Autodesk Inventor part; units mm, degrees
ref_plane "YZ Plane" through (0, 0, 0) normal (1, 0, 0) x (0, 1, 0)
ref_plane "XZ Plane" through (0, 0, 0) normal (0, 1, 0) x (-1, 0, 0)
ref_plane "XY Plane" through (0, 0, 0) normal (0, 0, 1) x (1, 0, 0)
sketch "Sketch1" plane through (0, 0, 0) normal (0, 0, 1) x (1, 0, 0)
  line L0 (0, -3.175) -> (31.75, -3.175)
  line L1 (31.75, -3.175) -> (31.75, -28.575)
  line L2 (31.75, -28.575) -> (0, -28.575)
  line L3 (0, -28.575) -> (0, -3.175)
  line L4 (0, -3.175) -> (5.715, -3.175)
  line L5 (5.715, -3.175) -> (5.715, 15.875)
  line L6 (5.715, 15.875) -> (0, 15.875)
  line L7 (0, 15.875) -> (0, -3.175)
  line L8 (26.035, -3.175) -> (31.75, -3.175)
  line L9 (31.75, -3.175) -> (31.75, 15.875)
  line L10 (31.75, 15.875) -> (26.035, 15.875)
  line L11 (26.035, 15.875) -> (26.035, -3.175)
  point P0 (0, 0)
  dimension "d0" = 25.4
  dimension "d1" = 5.715
  dimension "d2" = 5.715
  dimension "d3" = 19.05
  dimension "d4" = 31.75
  dimension "d24" = 20.32
extrude "Extrusion1" add sketch "Sketch1" against normal blind 15.875
sketch "Sketch2" plane through (0, 0, 0) normal (0, 0, 1) x (1, 0, 0)
  line L0 (31.75, -28.575) -> (0, -28.575)
  circle A0 centre (15.875, -15.875) radius 8.7439
  dimension "d10" = 17.4879
  dimension "d13" = 12.7
extrude "Extrusion2" cut sketch "Sketch2" against normal blind 15.875
sketch "Sketch3" plane through (31.75, -3.175, 0) normal (1, 0, 0) x (0, 0, -1)
  line L0 (0, 19.05) -> (15.875, 19.05)
  line L1 (-0.1272, 19.05) -> (15.7478, 19.05)
  circle A0 centre (7.9375, 12.7) radius 2.4447
  dimension "d16" = 4.8895
  dimension "d17" = 6.35
  dimension "d18" = 0
extrude "Extrusion3" cut sketch "Sketch3" against normal through all
fillet "Fillet1" radius 1.5875 2 edges at (5.715, -3.175, -7.9375) (26.035, -3.175, -7.9375)
fillet "Fillet3" radius 6.35 2 edges at (0, -28.575, -7.9375) (31.75, -28.575, -7.9375)
sketch "Sketch5" plane through (0, 0, 0) normal (0, 0, 1) x (1, 0, 0)
  line L0 (31.75, 15.875) -> (31.75, -22.225)
  line L1 (0, -22.225) -> (0, 15.875)
  line L2 (0, -22.2885) -> (3.175, -22.2885)
  line L3 (3.175, -22.2885) -> (3.175, -9.4615)
  line L4 (3.175, -9.4615) -> (0, -9.4615)
  line L5 (0, -9.4615) -> (0, -22.2885)
  line L6 (31.75, -9.4615) -> (28.575, -9.4615)
  line L7 (28.575, -9.4615) -> (28.575, -22.2885)
  line L8 (28.575, -22.2885) -> (31.75, -22.2885)
  line L9 (31.75, -22.2885) -> (31.75, -9.4615)
  circle A0 centre (15.875, -15.875) radius 8.7439
  point P0 (0, 0)
  point P1 (3.175, -15.875)
  dimension "d33" = 12.827
  dimension "d34" = 3.175
  dimension "d35" = 3.175
  dimension "d41" = 0
extrude "Extrusion5" cut sketch "Sketch5" against normal blind 25.4 contours L0 L9 L8 L7 L6 | L1 L4 L3 L2 L5
sketch "Sketch6" plane through (0, 0, 0) normal (0, 0, 1) x (1, 0, 0)
  line L0 (0, -9.4615) -> (0, 15.875)
  line L1 (0, -9.4615) -> (3.175, -9.4615)
  circle A0 centre (2.8575, 3.2385) radius 1.5875
  circle A1 centre (28.8925, 3.2385) radius 1.5875
  line L2 (28.575, -9.4615) -> (31.75, -9.4615)
  line L3 (26.035, -1.5875) -> (26.035, 15.875)
  point P0 (0, 0)
  dimension "d42" = 3.175
  dimension "d43" = 2.8575
  dimension "d44" = 12.7
  dimension "d45" = 3.175
  dimension "d50" = 12.7
  dimension "d51" = 2.8575
extrude "Extrusion6" cut sketch "Sketch6" against normal blind 25.4
properties part number "Smaller Needle Bearing Mount" material "Polyethylene, High Density"
Here's how the part is built. I have some questions about the finished solid (model axes, mm). A direction names the side the tool comes from. Give positions to 0.01 mm unless a question says otherwise; leave off trailing zeros. Write each loop counter-clockwise with the first axis right and the second up, starting at its lowest first coordinate (ties: lowest second). Pieces come first, ordered by that corner, then holes.
(1) If I drill on L1, parallel to X at y = 9, z = -11 (3 decimals); L2, parallel to Y at x = 29, z = -9.25 (1 decimal); L3, parallel to X at y = -13, z = -12 (3 decimals), over which ranges is the centre line in solid material (lowest first)?
Output values:
L1: x = 0 to 5.715, 26.035 to 31.75
L2: y = -27.5 to -22.3, -9.5 to 1.7, 4.8 to 7.5, 11.6 to 15.9
L3: x = 3.175 to 7.617, 24.133 to 28.575
(2) Imagine slicing it at D-D, the plane y = 4. Write out the boundary of the cut face in (x, z) (3 decimals), and give its area (3 significant figures).
Output values:
outline: (0, -15.875) - (1.465, -15.875) - (1.465, 0) - (0, 0) - close; (4.25, -15.875) - (5.715, -15.875) - (5.715, 0) - (4.25, 0) - close; (26.035, -15.875) - (27.5, -15.875) - (27.5, 0) - (26.035, 0) - close; (30.285, -15.875) - (31.75, -15.875) - (31.75, 0) - (30.285, 0) - close
area: 93.0 mm2
(3) Imagine slicing it at A-A, the plane y = -1. Write out the boundary of the cut face in (x, z) (3 decimals), and give its area (3 significant figures).
Output values:
outline: (0, -15.875) - (5.715, -15.875) - (5.715, 0) - (0, 0) - close; (26.035, -15.875) - (31.75, -15.875) - (31.75, 0) - (26.035, 0) - close
area: 181 mm2
(4) On a 3-axis mill with a long thin cutter (end or side, diameter ignored), from which of +Z, -Z, +X, -X, +Y, -Y can I reach the whole of each face in a straight line? I mean faces 4 (the face through (6.19, -2.72, -8.05)), 5 (the face through (3.175, -16, -8)), 6 (the face through (28.575, -16, -8)). Say none if no direction works.
Output values:
face 4: +Z, -Z, +Y
face 5: +Z, -Z, -X
face 6: +Z, -Z, +X
(5) Will these pins go through, and if not, where does the flat tip stop? pin 1 (4 mm diameter, centred on y = -12.5, z = -4.5, fed in from -X) (3 decimals); pin 2 (6.5 mm diameter, centred on y = -14.5, z = -10, fed in from +X) (3 decimals); pin 3 (2.5 mm diameter, centred on x = 2, z = -4.5, fed in from -Y).
Output values:
pin 1: stops at x = 3.175
pin 2: stops at x = 28.575
pin 3: stops at y = -27.77
(6) Thinking about a two-plate mould opening in X: for faces 1 (the face through (1.932, -26.786, -8.049)), 2 (the face through (2, -22.288, -8)), 3 (the face through (2.51, 1.69, -7.83)), which applies, pulls with the +X half, pulls with the -X half, needs draft (parallel to the pull), parting line crosses it, or undercut?
Output values:
face 1: pulls with the -X half
face 2: needs draft
face 3: undercut
(7) Imagine slicing it at C-C, the plane z = -6.5. Count the separate pieces of the cut face and the enclosed holes in it, and give its area (3 significant figures).
Output values:
separate pieces: 3
enclosed holes: 3
area: 625 mm2
(8) Imagine slicing it at B-B, the plane x = 2. Write out the boundary of the cut face in (y, z) (1 decimal).
Output values:
outline: (-26.9, -15.9) - (-22.3, -15.9) - (-22.3, 0) - (-26.9, 0) - close; (-9.5, -15.9) - (1.9, -15.9) - (1.9, 0) - (-9.5, 0) - close; (4.6, -15.9) - (15.9, -15.9) - (15.9, 0) - (4.6, 0) - close; hole circle Ø4.9 at (9.5, -7.9)
